from build123d import *

# Parameters (mm, degrees)
F0_R      = 9
F1_DEPTH  = 45
F2_R      = 4.5
F3_DEPTH  = 25
F6_DEPTH  = 25
F7_R      = 1.75
F8_DEPTH  = 7.5
F9_R      = 0.5
F10_R     = 0.5
F11_DEPTH = 32
F12_DEPTH = 32.36752
F13_DEPTH = 35.60573


with BuildPart() as f1:
    # F0 (on Top) → F1 (new body)
    with BuildSketch(Plane.XY):
        Circle(F0_R)
    extrude(amount=F1_DEPTH)

    # F2 (on face) → F3 (join)
    with BuildSketch(Plane.XY.offset(45)):
        Circle(F2_R)
    extrude(amount=F3_DEPTH)

    # F6 (add): a face of the model
    f6_faces = [f1.faces().sort_by_distance(p)[0] for p in [
        (0, 0, 70),
    ]]
    extrude(f6_faces, amount=F6_DEPTH)

    # F7 (on line) → F8 (join, symmetric)
    with BuildSketch(Plane(origin=(0, 0, 0), x_dir=(-1, 0, 0), z_dir=(0, 1, 0))):
        with Locations((0, 53.652189672)):
            Circle(F7_R)
    extrude(amount=F8_DEPTH, both=True)

    # F9
    f9_edges = [f1.edges().sort_by_distance(p)[0] for p in [
        (1.75, -7.5, 53.65219),
    ]]
    fillet(f9_edges, radius=F9_R)

    # F10
    f10_edges = [f1.edges().sort_by_distance(p)[0] for p in [
        (1.75, 7.5, 53.65219),
    ]]
    fillet(f10_edges, radius=F10_R)

    # F11 (add): a face of the model
    f11_faces = [f1.faces().sort_by_distance(p)[0] for p in [
        (0, 0, 95),
    ]]
    extrude(f11_faces, amount=-F11_DEPTH)

    # F12 (cut): a face of the model
    f12_faces = [f1.faces().sort_by_distance(p)[0] for p in [
        (0, 0, 95),
    ]]
    extrude(f12_faces, amount=-F12_DEPTH, mode=Mode.SUBTRACT)

    # F0 (on Top) → F13 (cut)
    with BuildSketch(Plane.XY):
        Circle(F0_R)
    extrude(amount=F13_DEPTH, mode=Mode.SUBTRACT)


solid = f1.part
Here's how the part is built. I have some questions about the finished solid (model axes, mm). A direction names the side the tool comes from. Give positions to 0.01 mm unless a question says otherwise; leave off trailing zeros. Order: outer loops, then holes, each group sorted by start corner. A loop starts at its lowest first (then second) coordinate and runs counter-clockwise, first axis right, second up. Notation, with made-up numbers: (10.5, 2.5) -> (68.5, 2.5) arc R19 cw to (68.5, 14.5) -> close; hole circle Ø2 at (-40, 7.5). An arc over 180 degrees is marked (long way). One line per item, written item: value. Start each with the question number.
1. Imagine slicing it at D-D, the plane z = 43. List the corners of the cut face in (x, y) for me, plus the area to 3 significant figures.
2. We'd pull the mould along Z, two halves only. Please class faces 1 (the face through (0, 0, 35.606)), 2 (the face through (0, 7.5, 54)), 3 (the face through (0.379, -5.553, 51.944)): released by +Z, released by -Z, zero draft, split by the parting line, or undercut.
3. For faces 4 (the face through (0, -7.5, 54)), 5 (the face through (0, 0, 62.632)), 6 (the face through (1.75, 5.59, 53.73)), which set-ups out of +Z, -Z, +X, -X, +Y, -Y let a thin tool reach every point of the face, with its end or its side?
4. I need wall thicknesses on probe 1 along Z at (x, y) = (2.25, -6); probe 2 along Y at (x, z) = (-1.75, 47.5); probe 3 along Y at (x, z) = (5.5, 41.75). Which ranges of each line are inside material? Lowest first, please. Write a range as from..to.
5. Imagine slicing it at C-C, the plane y = 5. List the corners of the cut face in (x, z) for me, plus the area to 3 significant figures.
6. Imagine slicing it at A-A, the plane y = 0. List the corners of the cut face in (x, z) for me, plus the area to 3 significant figures.
7. Imagine slicing it at B-B, the plane x = 0. List the corners of the cut face in (y, z) for me.
8. Will these pins go through, and if not, where does the flat tip stop? pin 1 Ø3 at (x, z) = (0, 53.5) entering from +Y; pin 2 Ø5 at (x, z) = (-5.5, 56) entering from +Y; pin 3 Ø2 at (x, z) = (0, 59.5) entering from +Y.
Values follow:
1. outline: circle Ø18 at (0, 0)
1. area: 254 mm2
2. face 1: released by -Z
2. face 2: zero draft
2. face 3: undercut
3. face 4: +Z, +X, -X, -Y
3. face 5: +Z, +X, -X, +Y, -Y
3. face 6: +Y
4. probe 1: z = 35.61..45
4. probe 2: y = -4.15..4.15
4. probe 3: y = -7.12..7.12
5. outline: (-7.48, 35.61) -> (7.48, 35.61) -> (7.48, 45) -> (-7.48, 45) -> close; circle Ø3.5 at (0, 53.65)
5. area: 150 mm2
6. outline: (-9, 35.61) -> (9, 35.61) -> (9, 45) -> (4.5, 45) -> (4.5, 62.63) -> (-4.5, 62.63) -> (-4.5, 45) -> (-9, 45) -> close
6. area: 328 mm2
7. outline: (-9, 35.61) -> (9, 35.61) -> (9, 45) -> (4.5, 45) -> (4.5, 51.9) -> (7, 51.9) arc R0.5 ccw to (7.5, 52.4) -> (7.5, 54.9) arc R0.5 ccw to (7, 55.4) -> (4.5, 55.4) -> (4.5, 62.63) -> (-4.5, 62.63) -> (-4.5, 55.4) -> (-7, 55.4) arc R0.5 ccw to (-7.5, 54.9) -> (-7.5, 52.4) arc R0.5 ccw to (-7, 51.9) -> (-4.5, 51.9) -> (-4.5, 45) -> (-9, 45) -> close
8. pin 1: stops at y = 7.5
8. pin 2: stops at y = 3.35
8. pin 3: stops at y = 4.5
